```python
from build123d import *

# Parameters (mm, degrees)
SKETCH1_W                  = 50
SKETCH1_H                  = 52.48
SKETCH1_R                  = 20.44
BOSS_EXTRUDE1_DEPTH        = 6.35
SKETCH4_R                  = 3.5
BOSS_EXTRUDE4_DEPTH        = 5
F_10_CLEARANCE_HOLE1_D     = 5.1054
F_10_CLEARANCE_HOLE1_DEPTH = 6.35
FILLET1_R                  = 6.35
CHAMFER1_SIZE              = 2
CHAMFER2_SIZE              = 2


with BuildPart() as part:
    # Sketch1 → Boss-Extrude1 (new body)
    with BuildSketch(Plane.XY):
        Rectangle(SKETCH1_W, SKETCH1_H)
        with Locations((0, 0.415)):
            Circle(SKETCH1_R, mode=Mode.SUBTRACT)
    extrude(amount=BOSS_EXTRUDE1_DEPTH)

    # Sketch4 → Boss-Extrude4 (add)
    with BuildSketch(Plane.XZ.offset(26.24)):
        Polygon((25, -44.5), (25, 0), (-25, 0), (-25, -44.5), (-39, -44.5), (-39, -63.5), (39, -63.5), (39, -44.5), align=None)
        with Locations((30, -54)):
            Circle(SKETCH4_R, mode=Mode.SUBTRACT)
        with Locations((-30, -54)):
            Circle(SKETCH4_R, mode=Mode.SUBTRACT)
    extrude(amount=-BOSS_EXTRUDE4_DEPTH)

    # #10 Clearance Hole1
    with Locations(Plane.XY.offset(6.35)):
        with Locations((17.960512242, -17.545512242), (-17.960512242, 18.375512242)):
            Hole(F_10_CLEARANCE_HOLE1_D / 2, depth=F_10_CLEARANCE_HOLE1_DEPTH)

    # Fillet1
    fillet1_edges = [part.edges().sort_by_distance(p)[0] for p in [
        (-25, -23.74, -44.5),
        (25, -23.74, -44.5),
    ]]
    fillet(fillet1_edges, radius=FILLET1_R)

    # Chamfer1
    chamfer1_edges = [part.edges().sort_by_distance(p)[0] for p in [
        (39, -23.74, -44.5),
        (39, -23.74, -63.5),
        (-39, -23.74, -63.5),
        (-39, -23.74, -44.5),
    ]]
    chamfer(chamfer1_edges, length=CHAMFER1_SIZE)

    # Chamfer2
    chamfer2_edges = [part.edges().sort_by_distance(p)[0] for p in [
        (-25, 26.24, 3.175),
        (25, 26.24, 3.175),
    ]]
    chamfer(chamfer2_edges, length=CHAMFER2_SIZE)


solid = part.part
```
Build history of the part. All positions in model axes, mm. A direction names the side the tool comes from. Coordinates: 2 decimals unless noted, no trailing zeros. Order: outer loops, then holes, each group sorted by start corner. A loop starts at its lowest first (then second) coordinate and runs counter-clockwise, first axis right, second up. Notation, with made-up numbers: (-30.5, -8.75) -> (-5.5, -8.75) arc R15 cw to (-5.5, 15.25) -> close; hole circle Ø9 at (3, -33.75). An arc over 180 degrees is marked (long way). Answer in a Markdown table with one row per item. Add a question column.
Q1. Drop flat-ended pins along their axis: pin 1 (13.5 mm diameter, centred on y = -1, z = -5.5, fed in from +X); pin 2 (14 mm diameter, centred on x = -5, y = 13.5, fed in from -Z); pin 3 (8 mm diameter, centred on x = -30, z = -54, fed in from +Y). Give the stop position or say it passes through.
Q2. Band-saw the part on D-D, the plane x = 28.5. List the corners of the cut face in (y, z).
Q3. Band-saw the part on B-B, the plane y = 3.5. List the corners of the cut face in (x, z), then the cut area to 3 significant figures.
Q4. Wall check: line 1 along Y through (x, z) = (0, 4) (3 decimals); line 2 along Y through (x, z) = (-22, -50); line 3 along Y through (x, z) = (-6.5, 1). Give the ranges that are in metal, low to high. Write a range as [from, to].
Q5. Band-saw the part on A-A, the plane x = 0. List the corners of the cut face in (y, z) (3 decimals).
Q6. Mould opens along Y. For faces 4 (the face through (18.293, -15.015, 3.131)), 5 (the face through (-23.99, 25.25, 3.13)), 6 (the face through (39, -24, -54)) say: +Y half, -Y half, draft (parallel to the pull), parting line (faces both ways), or undercut.
Q7. Which spindle directions (+Z, -Z, +X, -X, +Y, -Y) get a long thin tool onto all of the face, cutting with end or side? Do faces 1 (the face through (-34, -24, -44.5)), 2 (the face through (25, -10.5, 0.5)), 3 (the face through (-1, -21.24, -38)). Say none if no direction does.
Q8. Band-saw the part on C-C, the plane z = -25.5. List the corners of the cut face in (x, y), then the cut area to 3 significant figures.
Answers follow:
| question | item | result |
|---|---|---|
| 1 | pin 1 | x = 25 |
| 1 | pin 2 | z = 0 |
| 1 | pin 3 | y = -21.24 |
| 2 | outline | (-26.24, -63.5) -> (-21.24, -63.5) -> (-21.24, -57.16) -> (-26.24, -57.16) -> close; (-26.24, -50.84) -> (-21.24, -50.84) -> (-21.24, -43.82) -> (-26.24, -43.82) -> close |
| 3 | outline | (-25, 0) -> (-20.21, 0) -> (-20.21, 6.35) -> (-25, 6.35) -> close; (20.21, 0) -> (25, 0) -> (25, 6.35) -> (20.21, 6.35) -> close |
| 3 | area | 60.9 mm^2 |
| 4 | line 1 | [-26.24, -20.025], [20.855, 26.24] |
| 4 | line 2 | [-26.24, -21.24] |
| 4 | line 3 | [-26.24, -18.96], [19.79, 26.24] |
| 5 | outline | (-26.24, -63.5) -> (-21.24, -63.5) -> (-21.24, 0) -> (-20.025, 0) -> (-20.025, 6.35) -> (-26.24, 6.35) -> close; (20.855, 0) -> (26.24, 0) -> (26.24, 6.35) -> (20.855, 6.35) -> close |
| 6 | face 4 | undercut |
| 6 | face 5 | +Y half |
| 6 | face 6 | draft |
| 7 | face 1 | +Z, -X, +Y, -Y |
| 7 | face 2 | +Z, +X, +Y, -Y |
| 7 | face 3 | -Z, +X, -X, +Y |
| 8 | outline | (-25, -26.24) -> (25, -26.24) -> (25, -21.24) -> (-25, -21.24) -> close |
| 8 | area | 250 mm^2 |
